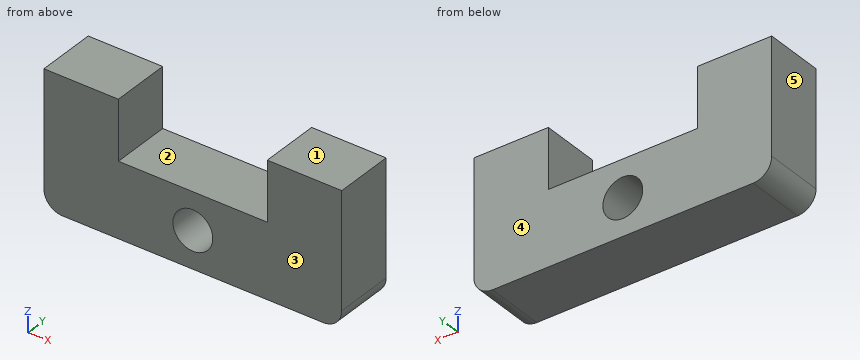
from build123d import *

# Parameters (mm, degrees)
SKETCH1_R           = 1.7
BOSS_EXTRUDE1_DEPTH = 5.08
FILLET1_R           = 1.5875


with BuildPart() as part:
    # Sketch1 → Boss-Extrude1 (new body)
    with BuildSketch(Plane(origin=(0, 0, 0), x_dir=(1, 0, 0), z_dir=(0, 1, 0))):
        Polygon((-12.7, -3.175), (-12.7, -8.255), (-6.35, -8.255), (-6.35, -3.175), (6.35, -3.175), (6.35, -8.255), (12.7, -8.255), (12.7, -3.175), (12.7, 3.175), (-12.7, 3.175), align=None)
        with Locations(Location((0, 0, 0), (0, 0, 270))):
            Circle(SKETCH1_R, mode=Mode.SUBTRACT)
    extrude(amount=BOSS_EXTRUDE1_DEPTH)

    # Fillet1
    fillet1_edges = [part.edges().sort_by_distance(p)[0] for p in [
        (-12.7, 2.54, -3.175),
        (12.7, 2.54, -3.175),
    ]]
    fillet(fillet1_edges, radius=FILLET1_R)


solid = part.part
Geometry check sheet. Reference: the model listing, model coordinates, mm. Face numbers are marked on the shaded views. A direction names the side the tool comes from. Give positions to 0.01 mm unless a question says otherwise; leave off trailing zeros. Order: outer loops, then holes, each group sorted by start corner. A loop starts at its lowest first (then second) coordinate and runs counter-clockwise, first axis right, second up.
1. Access from +Z, -Z, +X, -X, +Y, -Y to the whole of each face (thin tool, end or side, straight path). Record for the marked faces 1 and 2.
Completed:
face 1: +Z, +X, -X, +Y, -Y
face 2: +Z, +Y, -Y
2. Sectioned sample at B-B (x = 0). Record the boundary of the cut face in (y, z) (3 decimals), then the cut area to 3 significant figures.
Completed:
outline: (0, -3.175) - (5.08, -3.175) - (5.08, -1.7) - (0, -1.7) - close; (0, 1.7) - (5.08, 1.7) - (5.08, 3.175) - (0, 3.175) - close
area: 15.0 mm2
3. Depth check by flat-ended pin: pin 1 (2.5 mm diameter, centred on x = 0, z = 0, fed in from +Y); pin 2 (1.5 mm diameter, centred on x = 4.5, y = 4, fed in from +Z) (3 decimals). Enter the tip coordinate at first touch or a pass-through.
Completed:
pin 1: passes through
pin 2: stops at z = 3.175
4. Sectioned sample at A-A (z = 0). Record the boundary of the cut face in (x, y), then the cut area to 3 significant figures.
Completed:
outline: (-12.7, 0) - (-1.7, 0) - (-1.7, 5.08) - (-12.7, 5.08) - close; (1.7, 0) - (12.7, 0) - (12.7, 5.08) - (1.7, 5.08) - close
area: 112 mm2
5. Scan lines: line 1 (X direction, y = 3.7, z = 0); line 2 (X direction, y = 1.85, z = 5); line 3 (Z direction, x = -6, y = 0.55) (3 decimals). Record each from-to range of solid material in increasing order.
Completed:
line 1: x = -12.7 to -1.7, 1.7 to 12.7
line 2: x = -12.7 to -6.35, 6.35 to 12.7
line 3: z = -3.175 to 3.175
6. Draft check along Y on the marked faces 3, 4 and 5. Enter one of: pulls with the +Y half, pulls with the -Y half, needs draft (parallel to the pull), parting line crosses it, or undercut.
Completed:
face 3: pulls with the -Y half
face 4: pulls with the +Y half
face 5: needs draft
